Autodesk Inventor part; units mm, degrees
ref_plane "YZ Plane" through (0, 0, 0) normal (1, 0, 0) x (0, 1, 0)
ref_plane "XZ Plane" through (0, 0, 0) normal (0, 1, 0) x (-1, 0, 0)
ref_plane "XY Plane" through (0, 0, 0) normal (0, 0, 1) x (1, 0, 0)
sketch "Sketch1" plane through (0, 0, 0) normal (0, 0, 1) x (1, 0, 0)
  line L0 (-54.1531, -3.8255) -> (0, 29.3361)
  line L1 (0, 29.3361) -> (63.5, 30.9789)
  line L2 (-54.1531, -3.8255) -> (-46.1859, -16.836)
  line L3 (-46.1859, -16.836) -> (63.5, 18.2222)
  line L4 (63.5, 18.2222) -> (63.5, 30.9789)
  point P0 (0, 0)
  dimension "d0" = 150
  dimension "d1" = 63.5
  dimension "d2" = 63.5
extrude "Extrusion1" add sketch "Sketch1" along normal blind 25.4
fillet "Fillet1" radius 3.175 1 edges at (0, 29.3361, 12.7)
fillet "Fillet2" radius 3.175 1 edges at (63.5, 30.9789, 12.7)
fillet "Fillet3" radius 3.175 1 edges at (-54.1531, -3.8255, 12.7)
sketch "Sketch2" plane through (63.5, 18.2222, 0) normal (0.3045, -0.9525, 0) x (0.9525, 0.3045, 0)
  line L0 (-105.1746, 19.5706) -> (-8.2146, 19.5706)
  line L1 (-8.2146, 19.5706) -> (-8.2146, 4.4663)
  line L2 (-8.2146, 4.4663) -> (-105.1746, 4.4663)
  line L3 (-105.1746, 4.4663) -> (-105.1746, 19.5706)
  point P0 (-66.0333, 0)
extrude "Extrusion2" cut sketch "Sketch2" against normal blind 11.1125
CAD build for the part. Positions are in the model's coordinates, mm. A direction names the side the tool comes from. Round coordinates to 2 decimals unless told otherwise and drop trailing zeros. Loops run counter-clockwise (first coordinate to the right, second up) from the corner with the lowest first, then second, coordinate; pieces in that order, holes last. Notation, with made-up numbers: (78.25, 73) - (120.25, 73) arc R19 ccw to (120.25, 92) - close; hole circle Ø3 at (-37, -5). An arc over 180 degrees is marked (long way). Return JSON: item names as keys, results as strings. Group by question number.
Q1. Band-saw the part on B-B on x = 34. Give the cut face in (y, z).
Q2. Drill centre lines: line 1 along Z through (x, y) = (30.5, 11.5); line 2 along Y through (x, z) = (34, 12); line 3 along Y through (x, z) = (5, 7). Where is each one in solid material? Low to high. Write a range as [from, to].
Q3. Band-saw the part on C-C on z = 11.5. Give the cut face in (x, y) (3 decimals).
Q4. Band-saw the part on A-A on z = 22.5. Give the cut face in (x, y) (3 decimals), plus the area to 3 significant figures.
Q5. Two-plate mould, pull along Z, no slides. Class faces 1 (the face through (62.566, 29.97, 12.878)), 2 (the face through (7, 6, 19.571)), 3 (the face through (4, 13, 0)): +Z half, -Z half, draft (parallel to the pull), parting line (faces both ways), or undercut.
Q6. Tool access for faces 4 (the face through (7.89, 0.45, 4.06)), 5 (the face through (-38.35, -8.58, 11.91)), 6 (the face through (54.007, 20.94, 12.124)): list every direction of +Z, -Z, +X, -X, +Y, -Y with a clear straight run to the whole face (end or side of a thin tool).
Q7. Flat gauge pins, fed straight in: pin 1 Ø1 at (x, z) = (25.5, 19.5) entering from +Y; pin 2 Ø3 at (x, z) = (-13, 12.5) entering from -Y; pin 3 Ø4 at (x, z) = (-38, 6.5) entering from +Y. Where does each tip first touch, or does it go through?
Solutions:
{
 "1": {"outline": "(8.79, 0) - (30.22, 0) - (30.22, 25.4) - (8.79, 25.4) - (8.79, 19.57) - (20.46, 19.57) - (20.46, 4.47) - (8.79, 4.47) - close"},
 "2": {"line 1": "z = [0, 4.47], [19.57, 25.4]", "line 2": "y = [20.46, 30.22]", "line 3": "y = [11.19, 29.47]"},
 "3": {"outline": "(-52.495, -6.533) - (-46.186, -16.836) - (-36.682, -13.798) - (-40.064, -3.217) - (52.291, 26.308) - (55.675, 15.721) - (63.5, 18.222) - (63.5, 27.721) arc R3.175 ccw to (60.243, 30.895) - (0.85, 29.358) arc R3.175 ccw to (-0.726, 28.892) - (-51.445, -2.167) arc R3.175 ccw to start"},
 "4": {"outline": "(-52.495, -6.533) - (-46.186, -16.836) - (63.5, 18.222) - (63.5, 27.721) arc R3.175 ccw to (60.243, 30.895) - (0.85, 29.358) arc R3.175 ccw to (-0.726, 28.892) - (-51.445, -2.167) arc R3.175 ccw to start", "area": "2,610 mm^2"},
 "5": {"face 1": "draft", "face 2": "undercut", "face 3": "-Z half"},
 "6": {"face 4": "+Z, -Z, +X, -Y", "face 5": "+X", "face 6": "-Y"},
 "7": {"pin 1": "stops at y = 30.01", "pin 2": "stops at y = 4.96", "pin 3": "stops at y = 7.29"}
}
